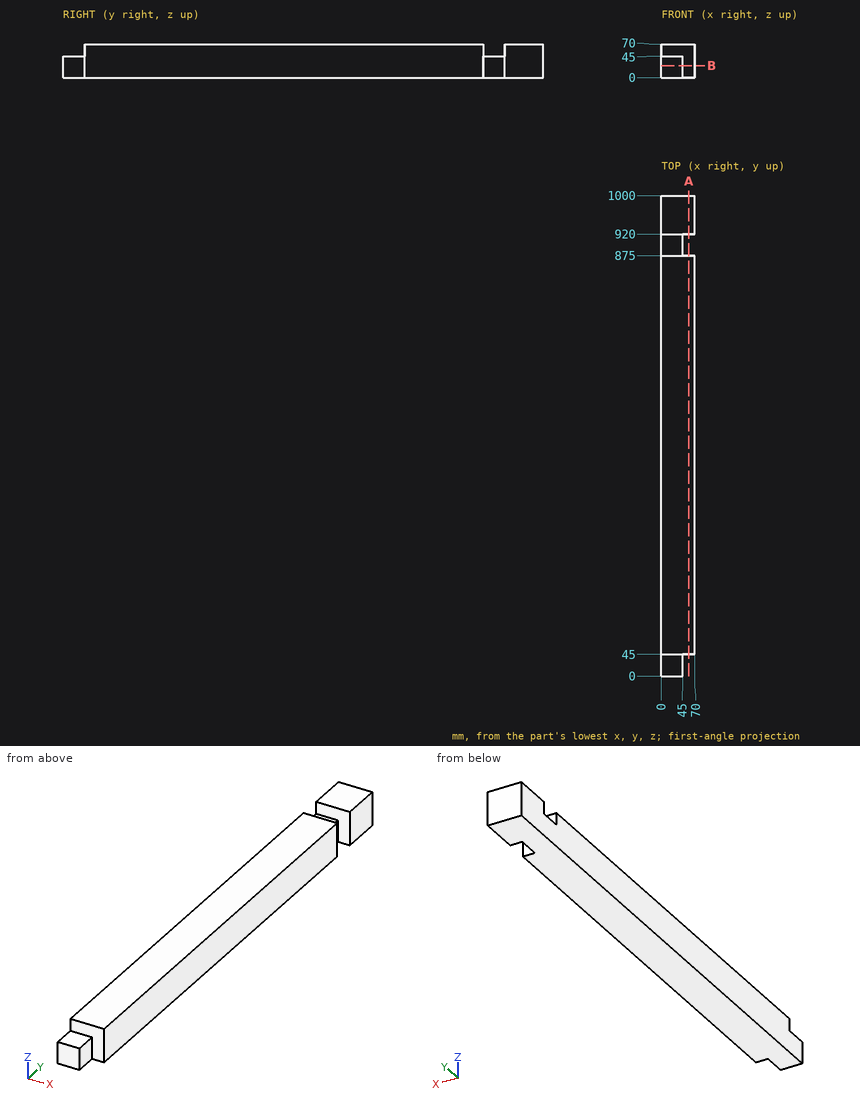
Could you check a few things on this drawing? It's one solid part, dimensions in mm from its lowest x, y, z. Round coordinates to 2 decimals unless told otherwise and drop trailing zeros. Loops run counter-clockwise (first coordinate to the right, second up) from the corner with the lowest first, then second, coordinate; pieces in that order, holes last.
Q1. Please list where these lines run through material, in increasing order: L1, parallel to Y at x = 58, z = 60; L2, parallel to Z at x = 30, y = 902.
Q2. I want a section at B-B (z = 25). Write out the boundary of the cut face in (x, y).
Q3. For P1, Ø22.5, axis at x = 15, y = 904.5, coming from the +Z side; P2, Ø10, axis at y = 673.5, z = 49, coming from the -X side; P3, Ø22.5, axis at y = 19, z = 26.5, coming from the +X side; P4, Ø1.5, axis at x = 56.5, z = 9, coming from the -Y side, each with a flat end and sliding along its axis, tell me the tip position at first contact or that it passes through.
Q4. I want a section at A-A (x = 57). Write out the boundary of the cut face in (y, z).
Answer below:
1. L1: y = 45 to 875, 920 to 1000
1. L2: z = 0 to 45
2. outline: (0, 0) - (45, 0) - (45, 45) - (70, 45) - (70, 875) - (45, 875) - (45, 920) - (70, 920) - (70, 1000) - (0, 1000) - close
3. P1: stops at z = 45
3. P2: stops at x = 0
3. P3: stops at x = 45
3. P4: stops at y = 45
4. outline: (45, 0) - (875, 0) - (875, 70) - (45, 70) - close; (920, 0) - (1000, 0) - (1000, 70) - (920, 70) - close
